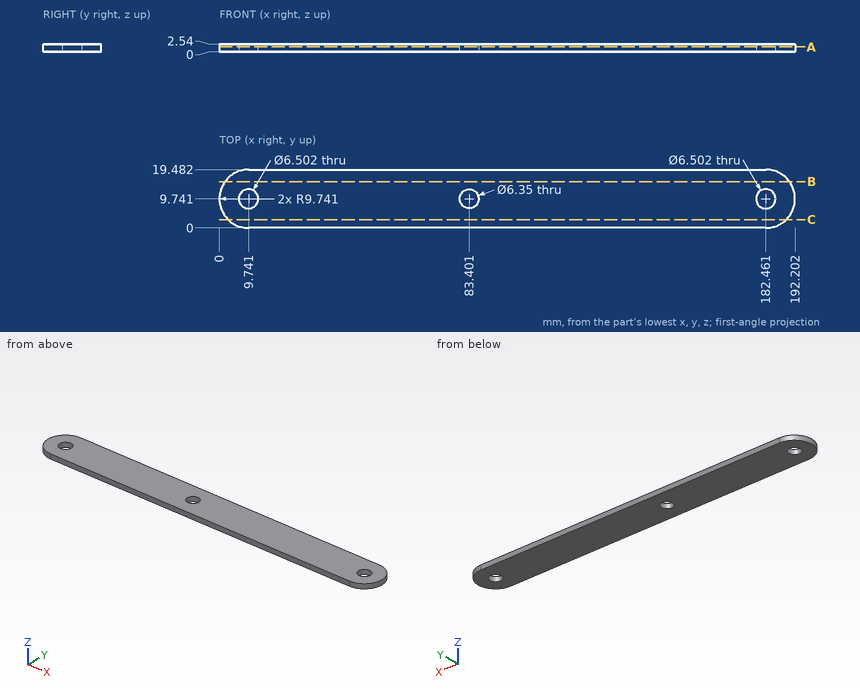
Source: three-view drawing plus pictorial views. Frame: mm from the lowest corner of the part. Round coordinates to 2 decimals unless told otherwise and drop trailing zeros. Write each loop counter-clockwise with the first axis right and the second up, starting at its lowest first coordinate (ties: lowest second). Pieces come first, ordered by that corner, then holes. Notation, with made-up numbers: (62.5, 11.25) -> (107.5, 11.25) arc R19 ccw to (107.5, 27.25) -> close; hole circle Ø11 at (-1.5, -8.5). An arc over 180 degrees is marked (long way). Return JSON: item names as keys, results as strings.
Q1. Section B-B on y = 15.5. Return the cut outline in (x, z) (1 decimal).
From the geometry:
{"outline": "(1.9, 0) -> (190.3, 0) -> (190.3, 2.5) -> (1.9, 2.5) -> close"}
Q2. Section C-C on y = 2.75. Return the cut outline in (x, z), and give its area (3 significant figures).
From the geometry:
{"outline": "(2.96, 0) -> (189.24, 0) -> (189.24, 2.54) -> (2.96, 2.54) -> close", "area": "473 mm2"}
Q3. Section A-A on z = 1.6. Give the number of separate pieces and of enclosed holes in the cut face, and give its area (4 significant figures).
From the geometry:
{"separate pieces": "1", "enclosed holes": "3", "area": "3,565 mm2"}
Q4. Ray query, line 1 (X direction, y = 8.5, z = 0.15) (1 decimal); line 2 (X direction, y = 12, z = 1.7) (1 decimal); line 3 (X direction, y = 13.5, z = 2.45) (1 decimal). Return the intervals inside material, ascending.
From the geometry:
{"line 1": "0.1 to 6.7, 12.7 to 80.5, 86.3 to 179.5, 185.5 to 192.1", "line 2": "0.3 to 7.4, 12.1 to 81.2, 85.6 to 180.1, 184.8 to 191.9", "line 3": "0.8 to 191.4"}
Q5. First-contact query: pin 1 Ø6 at (x, y) = (9.74, 9.74) entering from +Z; pin 2 Ø1.5 at (y, z) = (12.5, 1) entering from +X. Flat tips, straight axial feed; report the tip coordinate or a pass-through.
From the geometry:
{"pin 1": "through", "pin 2": "x = 191.99"}
